CAD build for the part. Positions are in the model's coordinates, mm. Give positions to 0.01 mm unless a question says otherwise; leave off trailing zeros. Order: outer loops, then holes, each group sorted by start corner. A loop starts at its lowest first (then second) coordinate and runs counter-clockwise, first axis right, second up.
```python
from build123d import *

# Parameters (mm, degrees)
SKETCH2_R           = 1.5
BOSS_EXTRUDE1_DEPTH = 4


with BuildPart() as part:
    # Sketch2 → Boss-Extrude1 (new body)
    with BuildSketch(Plane.XY):
        Polygon((-201.085, 510.519303279), (-148.79, -87.200696721), (148.79, -87.200696721), (201.085, 510.519303279), align=None)
        with Locations((-143.497000101, -21.490696721)):
            Circle(SKETCH2_R, mode=Mode.SUBTRACT)
        with Locations((-146.547451097, 13.376117712)):
            Circle(SKETCH2_R, mode=Mode.SUBTRACT)
        with Locations((-149.597902093, 48.242932145)):
            Circle(SKETCH2_R, mode=Mode.SUBTRACT)
        with Locations((-178.360333434, 376.989303279)):
            Circle(SKETCH2_R, mode=Mode.SUBTRACT)
        with Locations((-181.410784431, 411.856117712)):
            Circle(SKETCH2_R, mode=Mode.SUBTRACT)
        with Locations((-184.461235427, 446.722932145)):
            Circle(SKETCH2_R, mode=Mode.SUBTRACT)
        with Locations(Location((143.497000101, -21.490696721, 0), (0, 0, 180))):
            Circle(SKETCH2_R, mode=Mode.SUBTRACT)
        with Locations(Location((146.547451097, 13.376117712, 0), (0, 0, 180))):
            Circle(SKETCH2_R, mode=Mode.SUBTRACT)
        with Locations(Location((149.597902093, 48.242932145, 0), (0, 0, 180))):
            Circle(SKETCH2_R, mode=Mode.SUBTRACT)
        with Locations(Location((178.360333434, 376.989303279, 0), (0, 0, 180))):
            Circle(SKETCH2_R, mode=Mode.SUBTRACT)
        with Locations(Location((181.410784431, 411.856117712, 0), (0, 0, 180))):
            Circle(SKETCH2_R, mode=Mode.SUBTRACT)
        with Locations(Location((184.461235427, 446.722932145, 0), (0, 0, 180))):
            Circle(SKETCH2_R, mode=Mode.SUBTRACT)
    extrude(amount=BOSS_EXTRUDE1_DEPTH)


solid = part.part
```
Item 1: Slice it at A-A (z = 1.15). State how many separate pieces and enclosed holes the cut face has, and give its area (3 significant figures).
Item 2: Slice it at B-B (y = 394). Give the cut face in (x, z).
Item 3: Wall check: L1, parallel to X at y = 360.5, z = 3.6; L2, parallel to X at y = 136.5, z = 0.6. Give the ranges that are in metal, low to high.
Item 4: Drop a flat-ended pin along its axis: pin 1 Ø1 at (y, z) = (409.5, 2.5) entering from +X. Give the stop position or say it passes through.
Item 5: Slice it at C-C (y = 292). Give the cut face in (x, z).
A:
1. separate pieces: 1
1. enclosed holes: 12
1. area: 209,000 mm2
2. outline: (-190.89, 0) - (190.89, 0) - (190.89, 4) - (-190.89, 4) - close
3. L1: x = -187.96 to 187.96
3. L2: x = -168.36 to 168.36
4. pin 1: stops at x = 192.29
5. outline: (-181.97, 0) - (181.97, 0) - (181.97, 4) - (-181.97, 4) - close
